Drawing for the job (mm, zero at the part's lowest x, y, z). A direction names the side the tool comes from. Coordinates: 2 decimals unless noted, no trailing zeros. Loops run counter-clockwise (first coordinate to the right, second up) from the corner with the lowest first, then second, coordinate; pieces in that order, holes last. Notation, with made-up numbers: (-32, 71.25) -> (27, 71.25) arc R27 ccw to (27, 95.25) -> close; hole circle Ø6 at (12, 31.25). An arc over 180 degrees is marked (long way). Write item = value, one per line. Start each with the question number.
(1) Flat gauge pins, fed straight in: P1, Ø1, axis at x = 10.1, y = 8, coming from the -Z side; P2, Ø6.5, axis at x = 8, y = 8, coming from the +Z side; P3, Ø1, axis at y = 12, z = 1.5, coming from the -X side; P4, Ø3, axis at x = 12, z = 5, coming from the -Y side. Where does each tip first touch, or does it go through?
(2) Drill centre lines: line 1 (Y direction, x = 8, z = 2.5); line 2 (Y direction, x = 8, z = 1.4); line 3 (Z direction, x = 13, y = 12). Where is each one in solid material? Low to high. Write a range as from..to.
(3) Band-saw the part on C-C (x = 12). Write the cut outline in (y, z), and give its area (3 significant figures).
(4) Band-saw the part on A-A (x = 8). Write the cut outline in (y, z).
(5) Pull direction Z, two halves, no side cores. Call the marked faces 3, 4 and 5: +Z half, -Z half, draft (parallel to the pull), parting line (faces both ways), or undercut.
(6) Tool access for the marked faces 1 and 2: list every direction of +Z, -Z, +X, -X, +Y, -Y with a clear straight run to the whole face (end or side of a thin tool).
(7) Band-saw the part on D-D (y = 4.25). Write the cut outline in (x, z).
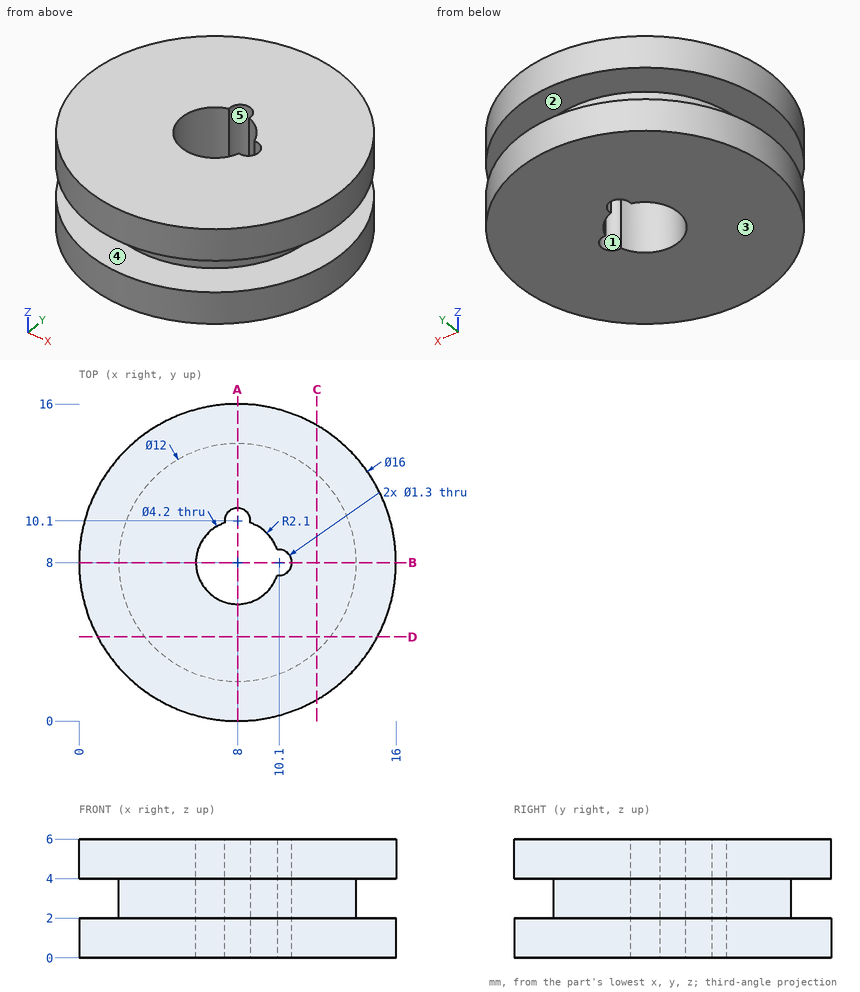
Findings below:
q1.P1 = through
q1.P2 = 6
q1.P3 = 0.81
q1.P4 = 0.4
q2.line_1 = 2..5.9, 10.75..14
q2.line_2 = 0..5.9, 10.75..16
q2.line_3 = 0..2, 4..6
q3.outline = (1.07, 0) -> (14.93, 0) -> (14.93, 2) -> (12.47, 2) -> (12.47, 4) -> (14.93, 4) -> (14.93, 6) -> (1.07, 6) -> (1.07, 4) -> (3.53, 4) -> (3.53, 2) -> (1.07, 2) -> close
q3.area = 73.3 mm²
q4.outline = (0, 0) -> (5.9, 0) -> (5.9, 6) -> (0, 6) -> (0, 4) -> (2, 4) -> (2, 2) -> (0, 2) -> close; (10.75, 0) -> (16, 0) -> (16, 2) -> (14, 2) -> (14, 4) -> (16, 4) -> (16, 6) -> (10.75, 6) -> close
q5.face_3 = -Z half
q5.face_4 = undercut
q5.face_5 = draft
q6.face_1 = +Z, -Z
q6.face_2 = none
q7.outline = (0.93, 0) -> (15.07, 0) -> (15.07, 2) -> (12.68, 2) -> (12.68, 4) -> (15.07, 4) -> (15.07, 6) -> (0.93, 6) -> (0.93, 4) -> (3.32, 4) -> (3.32, 2) -> (0.93, 2) -> close
